CAD build for the part. Positions are in the model's coordinates, mm. Give positions to 0.01 mm unless a question says otherwise; leave off trailing zeros. Order: outer loops, then holes, each group sorted by start corner. A loop starts at its lowest first (then second) coordinate and runs counter-clockwise, first axis right, second up.
Item 1: Band-saw the part on A-A on x = 151.5. Give the cut face in (y, z), plus the area to 3 significant figures.
Item 2: Band-saw the part on B-B on z = 63.5. Give the cut face in (x, y).
Item 3: Wall check: L1, parallel to Z at x = 30.5, y = 1513; L2, parallel to Z at x = 357, y = 1507; L3, parallel to X at y = 1514, z = -75.5. Give the ranges that are in metal, low to high.
Item 4: Flat gauge pin, fed straight in: P1, Ø3, axis at x = -148.31, z = -173.96, coming from the +Y side. Where does the tip first touch, or does it go through?
Item 5: Band-saw the part on C-C on y = 1510. Count the separate pieces of the cut face and the enclosed holes in it, plus the area to 3 significant figures.
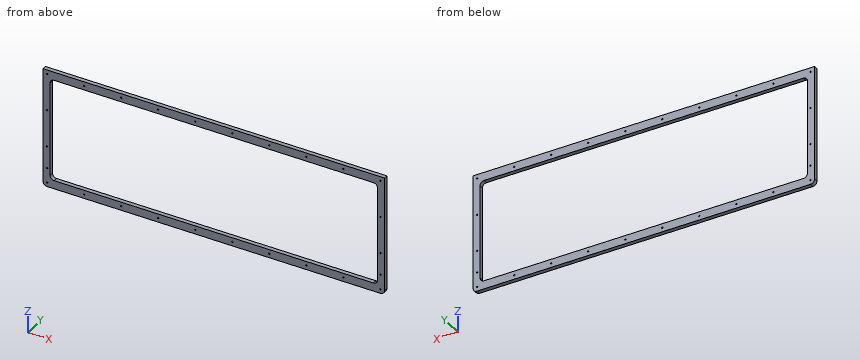
```python
from build123d import *

# Parameters (mm, degrees)
DODANIE_WYCI_GNI_CIE1_DEPTH = 10
WYTNIJ_WYCI_GNI_CIE1_DEPTH  = 10
SZKIC4_R                    = 1.55
WYTNIJ_WYCI_GNI_CIE2_DEPTH  = 10
SZYK_LINIOWY1_COUNT         = 9
SZYK_LINIOWY1_PITCH         = 89.555
SZYK_LINIOWY1_COL_COUNT     = 4
SZYK_LINIOWY1_COL_PITCH     = 89
SZKIC6_R                    = 1.55
WYTNIJ_WYCI_GNI_CIE3_DEPTH  = 10
SZYK_LINIOWY2_COUNT         = 4
SZYK_LINIOWY2_PITCH         = 89
SZYK_LINIOWY2_COL_COUNT     = 9
SZYK_LINIOWY2_COL_PITCH     = 89.555
SZYK_LINIOWY3_COUNT         = 2
SZYK_LINIOWY3_PITCH         = 36
SZYK_LINIOWY4_COUNT         = 2
SZYK_LINIOWY4_PITCH         = 231


with BuildPart() as part:
    # Szkic2 → Dodanie-wyciągnięcie1 (new body)
    with BuildSketch(Plane.ZX.offset(1505.947389818)):
        with BuildLine():
            Line((-183.955224703, 657.685033185), (-183.955224703, -148.314966815))
            ThreePointArc((-183.955224703, -148.314966815), (-181.026292515, -155.386034627), (-173.955224703, -158.314966815))
            Line((-173.955224703, -158.314966815), (103.044775297, -158.314966815))
            Line((103.044775297, -158.314966815), (103.044775297, 667.685033185))
            Line((103.044775297, 667.685033185), (-173.955224703, 667.685033185))
            ThreePointArc((-173.955224703, 667.685033185), (-181.026292515, 664.756100997), (-183.955224703, 657.685033185))
        make_face()
    extrude(amount=DODANIE_WYCI_GNI_CIE1_DEPTH)

    # Szkic3 → Wytnij-wyciągnięcie1 (cut)
    with BuildSketch(Plane(origin=(0, 1515.947389818, 0), x_dir=(1, 0, 0), z_dir=(0, 1, 0))):
        with BuildLine():
            Line((650.685033185, -73.044775297), (650.685033185, 153.955224703))
            ThreePointArc((650.685033185, 153.955224703), (647.756100997, 161.026292515), (640.685033185, 163.955224703))
            Line((640.685033185, 163.955224703), (-131.314966815, 163.955224703))
            ThreePointArc((-131.314966815, 163.955224703), (-138.386034627, 161.026292515), (-141.314966815, 153.955224703))
            Line((-141.314966815, 153.955224703), (-141.314966815, -73.044775297))
            ThreePointArc((-141.314966815, -73.044775297), (-138.386034627, -80.115843109), (-131.314966815, -83.044775297))
            Line((-131.314966815, -83.044775297), (640.685033185, -83.044775297))
            ThreePointArc((640.685033185, -83.044775297), (647.756100997, -80.115843109), (650.685033185, -73.044775297))
        make_face()
    extrude(amount=-WYTNIJ_WYCI_GNI_CIE1_DEPTH, mode=Mode.SUBTRACT)

    # Szkic4 → Wytnij-wyciągnięcie2 (cut)
    with BuildSketch(Plane(origin=(0, 1515.947389818, 0), x_dir=(1, 0, 0), z_dir=(0, 1, 0))):
        with Locations(Location((657.685033185, 173.955224703, 0), (0, 0, 270))):
            Circle(SZKIC4_R)
    wytnij_wyci_gni_cie2 = extrude(amount=-WYTNIJ_WYCI_GNI_CIE2_DEPTH, mode=Mode.SUBTRACT)

    # Szyk liniowy1: Wytnij-wyciągnięcie2 ×9
    with Locations(*[(-i * SZYK_LINIOWY1_PITCH, 0, 0) for i in range(1, SZYK_LINIOWY1_COUNT)]):
        add(wytnij_wyci_gni_cie2, mode=Mode.SUBTRACT)

    # Szyk liniowy1 col: Wytnij-wyciągnięcie2 ×4
    with Locations(*[(0, 0, i * SZYK_LINIOWY1_COL_PITCH) for i in range(1, SZYK_LINIOWY1_COL_COUNT)]):
        add(wytnij_wyci_gni_cie2, mode=Mode.SUBTRACT)

    # Szkic6 → Wytnij-wyciągnięcie3 (cut)
    with BuildSketch(Plane(origin=(0, 1515.947389818, 0), x_dir=(1, 0, 0), z_dir=(0, 1, 0))):
        with Locations(Location((-148.314966815, -93.044775297, 0), (0, 0, 270))):
            Circle(SZKIC6_R)
    wytnij_wyci_gni_cie3 = extrude(amount=-WYTNIJ_WYCI_GNI_CIE3_DEPTH, mode=Mode.SUBTRACT)

    # Szyk liniowy2: Wytnij-wyciągnięcie3 ×4
    with Locations(*[(0, 0, -i * SZYK_LINIOWY2_PITCH) for i in range(1, SZYK_LINIOWY2_COUNT)]):
        add(wytnij_wyci_gni_cie3, mode=Mode.SUBTRACT)

    # Szyk liniowy2 col: Wytnij-wyciągnięcie3 ×9
    with Locations(*[(i * SZYK_LINIOWY2_COL_PITCH, 0, 0) for i in range(1, SZYK_LINIOWY2_COL_COUNT)]):
        add(wytnij_wyci_gni_cie3, mode=Mode.SUBTRACT)

    # Szyk liniowy3: Wytnij-wyciągnięcie2 ×2
    with Locations(*[(0, 0, i * SZYK_LINIOWY3_PITCH) for i in range(1, SZYK_LINIOWY3_COUNT)]):
        add(wytnij_wyci_gni_cie2, mode=Mode.SUBTRACT)

    # Szyk liniowy4: Wytnij-wyciągnięcie3 ×2
    with Locations(*[(0, 0, -i * SZYK_LINIOWY4_PITCH) for i in range(1, SZYK_LINIOWY4_COUNT)]):
        add(wytnij_wyci_gni_cie3, mode=Mode.SUBTRACT)


solid = part.part
```
The answers:
1. outline: (1505.95, -183.96) - (1515.95, -183.96) - (1515.95, -163.96) - (1505.95, -163.96) - close; (1505.95, 83.04) - (1515.95, 83.04) - (1515.95, 103.04) - (1505.95, 103.04) - close
1. area: 400 mm2
2. outline: (-158.31, 1505.95) - (-141.31, 1505.95) - (-141.31, 1515.95) - (-158.31, 1515.95) - close; (650.69, 1505.95) - (667.69, 1505.95) - (667.69, 1515.95) - (650.69, 1515.95) - close
3. L1: z = -183.96 to -175.48, -172.43 to -163.96, 83.04 to 91.52, 94.57 to 103.04
3. L2: z = -183.96 to -163.96, 83.04 to 103.04
3. L3: x = -158.31 to -141.31, 650.69 to 667.69
4. P1: passes through
5. separate pieces: 1
5. enclosed holes: 27
5. area: 41,300 mm2
